```python
from build123d import *

# Parameters (mm, degrees)
F0_W     = 2.35
F0_H     = 14.5
F4_R     = 0.65
F5_DEPTH = 22.801
F6_W     = 11.5107307211
F6_H     = 11.4176999778
F6_R     = 3.9
F6_R_2   = 0.65
F7_DEPTH = 25


with BuildPart() as f1:
    # F0 (on Front) → F1 (revolve)
    with BuildSketch(Plane.XZ):
        Polygon((3.9, 11.4), (0, 11.4), (0, 3.1), (2.35, 3.1), (3.9, 3.1), align=None)
        with Locations((1.175, -4.15)):
            Rectangle(F0_W, F0_H)
    revolve(axis=Axis((0, 0, 0), (0, 0, -1)))

    # F2 (on Front) → F3 (revolve, cut)
    with BuildSketch(Plane.XZ):
        Polygon((2.05, -7.9), (2.35, -8.4), (2.35, -7.05), (2.05, -7.4), align=None)
        Polygon((2.35, -8.9), (1.2, -11.4), (2.35, -11.4), align=None)
    revolve(axis=Axis((0, 0, 0), (0, 0, -1)), mode=Mode.SUBTRACT)

    # F4 (on face) → F5 (cut, through all)
    with BuildSketch(Plane(origin=(0, 0, -11.4), x_dir=(1, 0, 0), z_dir=(0, 0, -1))):
        Circle(F4_R)
    extrude(amount=-F5_DEPTH, mode=Mode.SUBTRACT)

    # F6 (on face) → F7 (join)
    with BuildSketch(Plane.XY.offset(11.4)):
        Rectangle(F6_W, F6_H)
        Circle(F6_R, mode=Mode.SUBTRACT)
        Circle(F6_R)
        Circle(F6_R_2, mode=Mode.SUBTRACT)
    extrude(amount=F7_DEPTH)


solid = f1.part
```
Part model, mm, in its own coordinate system. A direction names the side the tool comes from. Round coordinates to 2 decimals unless told otherwise and drop trailing zeros. Loops run counter-clockwise (first coordinate to the right, second up) from the corner with the lowest first, then second, coordinate; pieces in that order, holes last.
Item 1: Mould opens along Z. For faces 3 (the face through (0, 5.709, 24)), 4 (the face through (-0.267, -2.033, -7.654)), 5 (the face through (0, 1, -11.4)) say: +Z half, -Z half, draft (parallel to the pull), parting line (faces both ways), or undercut.
Item 2: 3-axis set-ups, long thin cutter, end or side, ignore diameter. For faces 1 (the face through (-0.509, 2.294, -1.904)), 2 (the face through (5.755, 0, 24)): which of +Z, -Z, +X, -X, +Y, -Y reach the whole face in a straight line?
Item 3: Drop flat-ended pins along their axis: P1, Ø2, axis at x = 2.5, z = 9, coming from the -Y side; P2, Ø4, axis at x = 1, z = -0.5, coming from the +Y side. Give the stop position or say it passes through.
Item 4: Drill centre lines: line 1 (Y direction, x = 0, z = 10.5); line 2 (Y direction, x = 0, z = 17); line 3 (X direction, y = 0, z = 20.5). Where is each one in solid material? Low to high.
Item 5: Cut at D-D, the plane x = -3.25. Give the cut face in (y, z).
Item 6: Cut at B-B, the plane x = 0. Give the cut face in (y, z), then the cut area to 3 significant figures.
Item 7: Cut at C-C, the plane z = 7.5. Give the cut face in (x, y), then the cut area to 3 significant figures.
Item 8: Cut at A-A, the plane y = 0. Give the cut face in (x, z).
A:
1. face 3: draft
1. face 4: undercut
1. face 5: -Z half
2. face 1: -Z
2. face 2: +Z, -Z, +X, +Y, -Y
3. P1: stops at y = -3.6
3. P2: stops at y = 2.35
4. line 1: y = -3.9 to -0.65, 0.65 to 3.9
4. line 2: y = -5.71 to -0.65, 0.65 to 5.71
4. line 3: x = -5.76 to -0.65, 0.65 to 5.76
5. outline: (-5.71, 11.4) - (-2.16, 11.4) - (-2.16, 3.1) - (2.16, 3.1) - (2.16, 11.4) - (5.71, 11.4) - (5.71, 36.4) - (-5.71, 36.4) - close
6. outline: (-5.71, 11.4) - (-3.9, 11.4) - (-3.9, 3.1) - (-2.35, 3.1) - (-2.35, -7.05) - (-2.05, -7.4) - (-2.05, -7.9) - (-2.35, -8.4) - (-2.35, -8.9) - (-1.2, -11.4) - (-0.65, -11.4) - (-0.65, 36.4) - (-5.71, 36.4) - close; (0.65, -11.4) - (1.2, -11.4) - (2.35, -8.9) - (2.35, -8.4) - (2.05, -7.9) - (2.05, -7.4) - (2.35, -7.05) - (2.35, 3.1) - (3.9, 3.1) - (3.9, 11.4) - (5.71, 11.4) - (5.71, 36.4) - (0.65, 36.4) - close
6. area: 353 mm2
7. outline: circle Ø7.8 at (0, 0); hole circle Ø1.3 at (0, 0)
7. area: 46.5 mm2
8. outline: (-5.76, 11.4) - (-3.9, 11.4) - (-3.9, 3.1) - (-2.35, 3.1) - (-2.35, -7.05) - (-2.05, -7.4) - (-2.05, -7.9) - (-2.35, -8.4) - (-2.35, -8.9) - (-1.2, -11.4) - (-0.65, -11.4) - (-0.65, 36.4) - (-5.76, 36.4) - close; (0.65, -11.4) - (1.2, -11.4) - (2.35, -8.9) - (2.35, -8.4) - (2.05, -7.9) - (2.05, -7.4) - (2.35, -7.05) - (2.35, 3.1) - (3.9, 3.1) - (3.9, 11.4) - (5.76, 11.4) - (5.76, 36.4) - (0.65, 36.4) - close
